Verification items for the finished model (mm, model axes). A direction names the side the tool comes from. Coordinates: 2 decimals unless noted, no trailing zeros. Order: outer loops, then holes, each group sorted by start corner. A loop starts at its lowest first (then second) coordinate and runs counter-clockwise, first axis right, second up.
Q1. Set-up check for faces 1 (the flat face through (0, 0, 0)), 2 (the flat face through (5, 1, 2)): record each of +Z, -Z, +X, -X, +Y, -Y from which the full face is reachable in a straight line by a thin tool's end or side.
Q2. Cross-section at A-A, the plane y = 24. Record the boundary of the cut face in (x, z), and give its area (3 significant figures).
Q3. Thickness scan on line 1 (Y direction, x = 5.25, z = -3.5); line 2 (Z direction, x = -4, y = 125.5); line 3 (X direction, y = 96.5, z = -4.75). Record the ranges inside material, lowest first.
Q4. Cross-section at B-B, the plane x = 3.5. Record the boundary of the cut face in (y, z), and give its area (3 significant figures).
Q5. Depth check by flat-ended pin: P1, Ø6.5, axis at x = 3, z = 2, coming from the -Y side; P2, Ø3, axis at x = 2.5, y = 58, coming from the -Z side; P3, Ø1.5, axis at x = -1.5, y = 28, coming from the -Z side. Enter the tip coordinate at first touch or a pass-through.
Autodesk Inventor part; units mm, degrees
ref_plane "YZ Plane" through (0, 0, 0) normal (1, 0, 0) x (0, 1, 0)
ref_plane "XZ Plane" through (0, 0, 0) normal (0, 1, 0) x (-1, 0, 0)
ref_plane "XY Plane" through (0, 0, 0) normal (0, 0, 1) x (1, 0, 0)
sketch "Sketch1" plane through (0, 0, 0) normal (0, 1, 0) x (-1, 0, 0)
  line L0 (6.35, 3.6662) -> (6.35, -3.6662)
  line L1 (6.35, -3.6662) -> (0, -7.3323)
  line L2 (0, -7.3323) -> (-6.35, -3.6662)
  line L3 (-6.35, -3.6662) -> (-6.35, 3.6662)
  line L4 (-6.35, 3.6662) -> (0, 7.3323)
  line L5 (0, 7.3323) -> (6.35, 3.6662)
  point P0 (0, 0)
  point P1 (0, 0)
  dimension "d0" = 12.7
extrude "Extrusion1" add sketch "Sketch1" along normal blind 140
sketch "Sketch2" plane through (0, 0, 0) normal (0, 0, 1) x (1, 0, 0)
  line L0 (-15, 1) -> (-5, 1)
  line L1 (-5, 1) -> (-5, 2.5)
  line L2 (-5, 2.5) -> (-15, 2.5)
  line L3 (-15, 2.5) -> (-15, 1)
  line L4 (0, 0) -> (0, 140)
  line L5 (0, 0) -> (6.35, 0)
  line L6 (0, -26) -> (0, 156)
  line L7 (-15, 46) -> (-5, 46)
  line L8 (-5, 46) -> (-5, 47.5)
  line L9 (-5, 47.5) -> (-15, 47.5)
  line L10 (-15, 47.5) -> (-15, 46)
  point P0 (-15, 46.75)
  dimension "d3" = 1.5
  dimension "d4" = 10
  dimension "d5" = 5
  dimension "d6" = 1
  dimension "d8" = 43.5
revolve "Revolution1" cut sketch "Sketch2" angle 360 about axis through (0, -10, 0) along (0, 1, 0)
properties part number "Wasp Pivot Axle"
Check values:
1. face 1: +Z, -Z, +X, -X, -Y
1. face 2: none
2. outline: (-6.35, -3.67) - (0, -7.33) - (6.35, -3.67) - (6.35, 3.67) - (0, 7.33) - (-6.35, 3.67) - close
2. area: 140 mm2
3. line 1: y = 0 to 1, 2.5 to 46, 47.5 to 140
3. line 2: z = -5.02 to 5.02
3. line 3: x = -4.47 to 4.47
4. outline: (0, -5.31) - (1, -5.31) - (1, -3.57) - (2.5, -3.57) - (2.5, -5.31) - (46, -5.31) - (46, -3.57) - (47.5, -3.57) - (47.5, -5.31) - (140, -5.31) - (140, 5.31) - (47.5, 5.31) - (47.5, 3.57) - (46, 3.57) - (46, 5.31) - (2.5, 5.31) - (2.5, 3.57) - (1, 3.57) - (1, 5.31) - (0, 5.31) - close
4. area: 1,480 mm2
5. P1: stops at y = 0
5. P2: stops at z = -6.75
5. P3: stops at z = -6.9
